Check sheet for the drawn part. Datum: minimum x, y, z corner. Units: mm. A direction names the side the tool comes from. Give positions to 0.01 mm unless a question says otherwise; leave off trailing zeros. Order: outer loops, then holes, each group sorted by start corner. A loop starts at its lowest first (then second) coordinate and runs counter-clockwise, first axis right, second up. Notation, with made-up numbers: M 34,-31 L 70,-31 A28 ccw 70,7 Z; hole C -14,-11.75 d11. An arc over 180 degrees is marked long. Put each result on its own line as item: value. Start each with the question number.
Q1. Mould release check, pull along Y, two halves, no side actions. Record for the marked faces 3, 4 and 5: +Y half, -Y half, draft (parallel to the pull), parting line (faces both ways), or undercut.
Q2. Section check A-A on y = 11.5. Record the cut outline in (x, z) (1 decimal).
Q3. Go/stop test with a flat-tipped pin: pin 1 (1 mm diameter, centred on x = 11, z = 2, fed in from -Y) (1 decimal). Record where the tip stops, or that it passes through.
Q4. Section check B-B on x = 8. Record the cut outline in (y, z).
Q5. Access from +Z, -Z, +X, -X, +Y, -Y to the whole of each face (thin tool, end or side, straight path). Record for the marked faces 1 and 2.
Q6. Material ranges on L1, parallel to Y at x = 7.25, z = 0.35; L2, parallel to X at y = 14.25, z = 1.7; L3, parallel to Y at x = 10, z = 0.3, recorded low to high.
Q7. Section check C-C on z = 0.95. Record the cut outline in (x, y) (1 decimal).
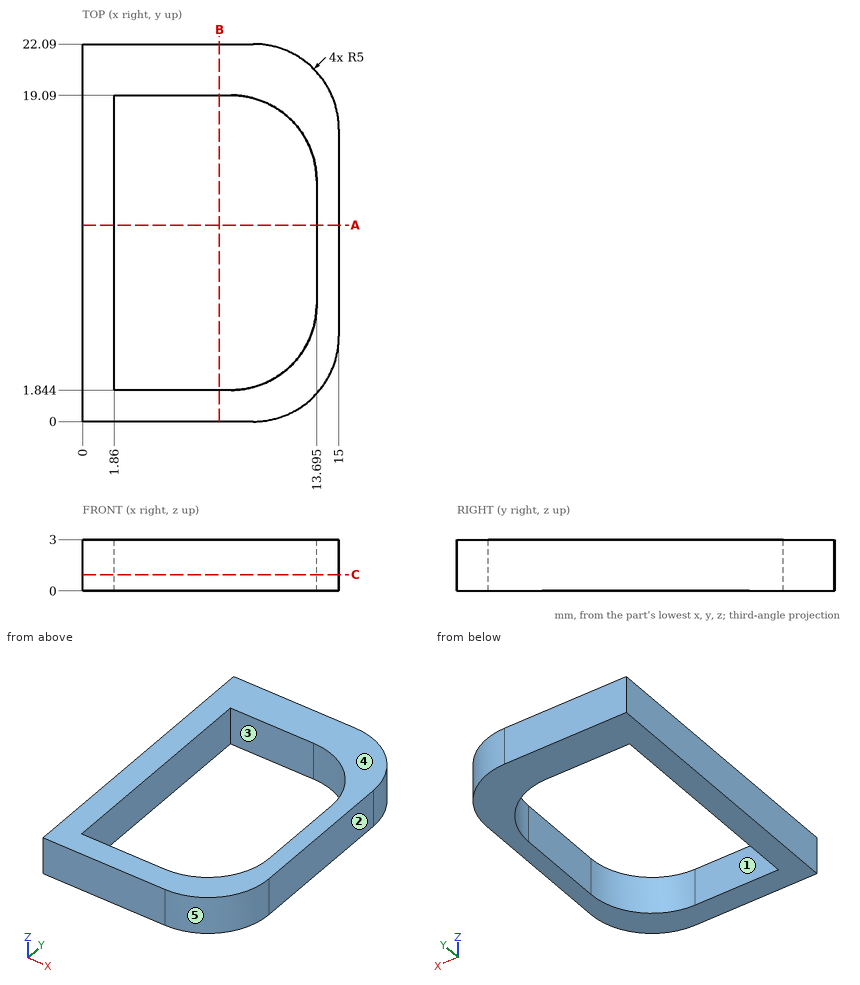
Results found:
1. face 3: undercut
1. face 4: draft
1. face 5: -Y half
2. outline: M 0,0 L 1.9,0 L 1.9,3 L 0,3 Z; M 13.7,0 L 15,0 L 15,3 L 13.7,3 Z
3. pin 1: stops at y = 0
4. outline: M 0,0 L 1.84,0 L 1.84,3 L 0,3 Z; M 19.09,0 L 22.09,0 L 22.09,3 L 19.09,3 Z
5. face 1: +Z, -Z
5. face 2: +Z, -Z, +X, +Y, -Y
6. L1: y = 0 to 1.84, 19.09 to 22.09
6. L2: x = 0 to 1.86, 13.69 to 15
6. L3: y = 0 to 2.02, 18.92 to 22.09
7. outline: M 0,0 L 10,0 A5 ccw 15,5 L 15,17.1 A5 ccw 10,22.1 L 0,22.1 Z; hole M 1.9,1.8 L 8.7,1.8 A5 ccw 13.7,6.8 L 13.7,14.1 A5 ccw 8.7,19.1 L 1.9,19.1 Z
